```python
from build123d import *

# Parameters (mm, degrees)
F1_DEPTH  = 8.6
F3_DEPTH  = 7.7
F5_DEPTH  = 5
F6_W      = 45.6
F6_H      = 8.6
F7_DEPTH  = 3
F8_W      = 5.6
F8_H      = 35
F9_DEPTH  = 14.2
F10_W     = 45.6
F10_H     = 8.6
F11_DEPTH = 3
F13_DEPTH = 5
F15_DEPTH = 2


with BuildPart() as f1:
    # F0 (on Front) → F1 (new body)
    with BuildSketch(Plane.XZ):
        with BuildLine():
            Line((3.4848013847, 64.4517231077), (-42.1151986153, 64.4517231077))
            ThreePointArc((-42.1151986153, 64.4517231077), (-48.479159646, 61.8156841384), (-51.1151986153, 55.4517231077))
            Line((-51.1151986153, 55.4517231077), (-51.1151986153, -55.3482768923))
            ThreePointArc((-51.1151986153, -55.3482768923), (-48.479159646, -61.712237923), (-42.1151986153, -64.3482768923))
            Line((-42.1151986153, -64.3482768923), (3.4848013847, -64.3482768923))
            ThreePointArc((3.4848013847, -64.3482768923), (9.8487624154, -61.712237923), (12.4848013847, -55.3482768923))
            Line((12.4848013847, -55.3482768923), (12.4848013847, 55.4517231077))
            ThreePointArc((12.4848013847, 55.4517231077), (9.8487624154, 61.8156841384), (3.4848013847, 64.4517231077))
        make_face()
    extrude(amount=F1_DEPTH)

    # F2 (on face) → F3 (cut)
    with BuildSketch(Plane.XZ.offset(8.6)):
        with BuildLine():
            Line((0.9848013847, 61.9517231077), (-39.6151986153, 61.9517231077))
            ThreePointArc((-39.6151986153, 61.9517231077), (-45.979159646, 59.3156841384), (-48.6151986153, 52.9517231077))
            Line((-48.6151986153, 52.9517231077), (-48.6151986153, -52.8482768923))
            ThreePointArc((-48.6151986153, -52.8482768923), (-45.979159646, -59.212237923), (-39.6151986153, -61.8482768923))
            Line((-39.6151986153, -61.8482768923), (0.9848013847, -61.8482768923))
            ThreePointArc((0.9848013847, -61.8482768923), (7.3487624154, -59.212237923), (9.9848013847, -52.8482768923))
            Line((9.9848013847, -52.8482768923), (9.9848013847, 52.9517231077))
            ThreePointArc((9.9848013847, 52.9517231077), (7.3487624154, 59.3156841384), (0.9848013847, 61.9517231077))
        make_face()
    extrude(amount=-F3_DEPTH, mode=Mode.SUBTRACT)

    # F4 (on face) → F5 (cut)
    with BuildSketch(Plane(origin=(0, 0, 0), x_dir=(-1, 0, 0), z_dir=(0, 1, 0))):
        with BuildLine():
            Line((6.0151986153, 60.4517231077), (-2.9848013847, 60.4517231077))
            ThreePointArc((-2.9848013847, 60.4517231077), (-6.1667819, 59.133703623), (-7.4848013847, 55.9517231077))
            ThreePointArc((-7.4848013847, 55.9517231077), (-6.1667819, 52.7697425924), (-2.9848013847, 51.4517231077))
            Line((-2.9848013847, 51.4517231077), (6.0151986153, 51.4517231077))
            ThreePointArc((6.0151986153, 51.4517231077), (9.1971791307, 52.7697425924), (10.5151986153, 55.9517231077))
            ThreePointArc((10.5151986153, 55.9517231077), (9.1971791307, 59.133703623), (6.0151986153, 60.4517231077))
        make_face()
    extrude(amount=-F5_DEPTH, mode=Mode.SUBTRACT)

    # F6 (on face) → F7 (cut)
    with BuildSketch(Plane(origin=(0, 0, -64.3482768923), x_dir=(1, 0, 0), z_dir=(0, 0, -1))):
        with Locations((-19.3151986153, 4.3)):
            Rectangle(F6_W, F6_H)
    extrude(amount=-F7_DEPTH, mode=Mode.SUBTRACT)

    # F8 (on face) → F9 (cut)
    with BuildSketch(Plane(origin=(-51.1151986153, 0, 0), x_dir=(0, -1, 0), z_dir=(-1, 0, 0))):
        with Locations((4.3, 32.9517231077)):
            Rectangle(F8_W, F8_H)
    extrude(amount=-F9_DEPTH, mode=Mode.SUBTRACT)

    # F10 (on face) → F11 (cut)
    with BuildSketch(Plane.XY.offset(64.4517231077)):
        with Locations((-19.3151986153, -4.3)):
            Rectangle(F10_W, F10_H)
    extrude(amount=-F11_DEPTH, mode=Mode.SUBTRACT)

    # F12 (on face) → F13 (join)
    with BuildSketch(Plane(origin=(0, 0, 0), x_dir=(-1, 0, 0), z_dir=(0, 1, 0))):
        Polygon((10.6879380899, 31.2634583622), (6.749325754, 31.2634583622), (3.9166819364, 27.1432485372), (7.8552942723, 27.1432485372), align=None)
        Polygon((13.5205856233, 27.1432485372), (10.6879380899, 31.2634583622), (7.8552942723, 27.1432485372), align=None)
        Polygon((16.3532294408, 31.2634583622), (10.6879380899, 31.2634583622), (13.5205856233, 27.1432485372), align=None)
        Polygon((7.8552942723, 27.1432485372), (3.9166819364, 27.1432485372), (17.0616876136, 8.9319211103), align=None)
        Polygon((19.2072947722, 27.1432485372), (16.3532294408, 31.2634583622), (13.5205856233, 27.1432485372), align=None)
        Polygon((22.0399385898, 31.2634583622), (16.3532294408, 31.2634583622), (19.2072947722, 27.1432485372), align=None)
        Polygon((13.5205856233, 27.1432485372), (7.8552942723, 27.1432485372), (17.0616876136, 8.9319211103), align=None)
        Polygon((19.2072947722, 27.1432485372), (13.5205856233, 27.1432485372), (17.0616876136, 8.9319211103), align=None)
        Polygon((24.8940039212, 27.1432485372), (17.0616876136, 8.9319211103), (29.5819732873, 27.1432485372), align=None)
        Polygon((19.2072947722, 27.1432485372), (17.0616876136, 8.9319211103), (24.8940039212, 27.1432485372), align=None)
        Polygon((24.8940039212, 27.1432485372), (22.0399385898, 31.2634583622), (19.2072947722, 27.1432485372), align=None)
        Polygon((26.749325754, 31.2634583622), (22.0399385898, 31.2634583622), (24.8940039212, 27.1432485372), (29.5819732873, 27.1432485372), align=None)
    extrude(amount=F13_DEPTH)

    # F14 (on face) → F15 (join)
    with BuildSketch(Plane(origin=(0, 5, 0), x_dir=(-1, 0, 0), z_dir=(0, 1, 0))):
        Polygon((12.4146133892, 31.2634583622), (9.5819695716, 27.1432485372), (15.2472572067, 27.1432485372), align=None)
        Polygon((15.2472572067, 27.1432485372), (9.5819695716, 27.1432485372), (17.0616876136, 8.9319211103), align=None)
        Polygon((16.749325754, 31.2634583622), (15.2472572067, 27.1432485372), (18.2513943012, 27.1432485372), align=None)
        Polygon((18.2513943012, 27.1432485372), (15.2472572067, 27.1432485372), (17.0616876136, 8.9319211103), align=None)
        Polygon((18.2513943012, 27.1432485372), (17.0616876136, 8.9319211103), (23.9166819364, 27.1432485372), align=None)
        Polygon((21.0840381188, 31.2634583622), (18.2513943012, 27.1432485372), (23.9166819364, 27.1432485372), align=None)
    extrude(amount=F15_DEPTH)


solid = f1.part
```
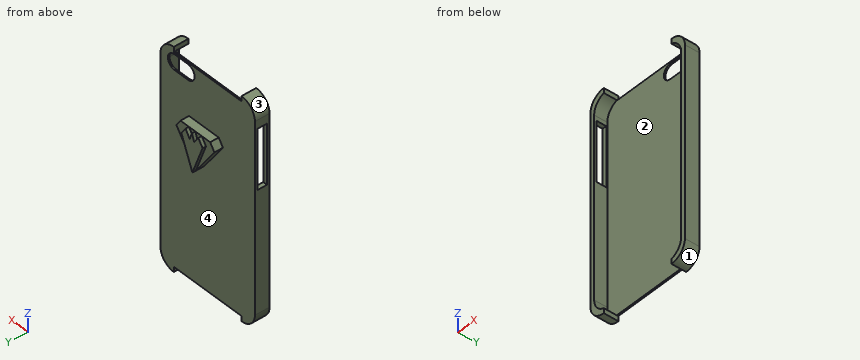
For this review, take the finished solid that the model builds, in its own axes (mm). Face numbers are marked on the shaded views. Coordinates: 2 decimals unless noted, no trailing zeros. Loops run counter-clockwise (first coordinate to the right, second up) from the corner with the lowest first, then second, coordinate; pieces in that order, holes last.
1. Add section C-C, the plane z = 19. Give the boundary of the cut face in (x, y), then the cut area to 3 significant figures.
2. Insertion check: P1, Ø0.8, axis at x = -50, z = 35, coming from the +Y side; P2, Ø3.5, axis at y = -4, z = 63.5, coming from the -X side; P3, Ø3, axis at y = 3.5, z = 23.5, coming from the +X side; P4, Ø4, axis at x = -31.5, y = -4.5, coming from the -Z side. Each pin has a flat end and moves straight along its axis. Give the tip position at first contact, or say it passes through.
3. Add section B-B, the plane y = -4. Give the boundary of the cut face in (x, z), then the cut area to 3 significant figures.
4. Add section D-D, the plane y = 3.5. Give the boundary of the cut face in (x, z), then the cut area to 3 significant figures.
5. For line 1 (X direction, y = -6.5, z = -4); line 2 (Y direction, x = -5, z = 2.5); line 3 (Z direction, x = -15, y = -0.25), list the stretches that pass through material, from the lowest coordinate up.
6. Add section A-A, the plane z = -39. Give the boundary of the cut face in (x, y).
7. Mouldability with a two-part tool opening along Z and no side actions: class the marked faces 1, 2, 3 and 4 as +Z half, -Z half, draft (parallel to the pull), parting line (faces both ways), or undercut.
Result:
1. outline: (-51.12, -8.6) - (-48.62, -8.6) - (-48.62, -7.1) - (-51.12, -7.1) - close; (-51.12, -1.5) - (-48.62, -1.5) - (-48.62, -0.9) - (9.98, -0.9) - (9.98, -8.6) - (12.48, -8.6) - (12.48, 0) - (-9.79, 0) - (-9.79, 5) - (-12.93, 5) - (-12.93, 7) - (-20.85, 7) - (-20.85, 5) - (-23.98, 5) - (-23.98, 0) - (-51.12, 0) - close
1. area: 169 mm2
2. P1: stops at y = 0
2. P2: stops at x = -48.54
2. P3: stops at x = -5.46
2. P4: passes through
3. outline: (-51.12, -55.35) arc R9 ccw to (-42.12, -64.35) - (-42.12, -61.49) arc R9 cw to (-48.62, -52.85) - (-48.62, 15.45) - (-51.12, 15.45) - close; (-51.12, 50.45) - (-48.62, 50.45) - (-48.62, 52.95) arc R9 cw to (-42.12, 61.6) - (-42.12, 64.45) arc R9 ccw to (-51.12, 55.45) - close; (3.48, -64.35) arc R9 ccw to (12.48, -55.35) - (12.48, 55.45) arc R9 ccw to (3.48, 64.45) - (3.48, 61.6) arc R9 cw to (9.98, 52.95) - (9.98, -52.85) arc R9 cw to (3.48, -61.49) - close
3. area: 620 mm2
4. outline: (-29.58, 27.14) - (-17.06, 8.93) - (-3.92, 27.14) - (-6.75, 31.26) - (-26.75, 31.26) - close
4. area: 328 mm2
5. line 1: x = -51.12 to -48.62, 9.98 to 12.48
5. line 2: y = -0.9 to 0
5. line 3: z = -61.35 to 61.45
6. outline: (-51.12, -8.6) - (-48.62, -8.6) - (-48.62, -0.9) - (9.98, -0.9) - (9.98, -8.6) - (12.48, -8.6) - (12.48, 0) - (-51.12, 0) - close
7. face 1: -Z half
7. face 2: undercut
7. face 3: +Z half
7. face 4: draft
